Input: part model. Units: mm. Frame: model coordinates. Coordinates: 2 decimals unless noted, no trailing zeros. Write each loop counter-clockwise with the first axis right and the second up, starting at its lowest first coordinate (ties: lowest second). Pieces come first, ordered by that corner, then holes. Notation, with made-up numbers: M 80.25,-32 L 99.25,-32 A21 cw 99.25,-24 Z; hole C -5.75,-21 d3. An arc over 180 degrees is marked long. Answer as a JSON object with one key per item and string values. Group by question number.
from build123d import *

# Parameters (mm, degrees)
BOSS_EXTRUDE1_DEPTH = 5
SKETCH4_W           = 27
SKETCH4_H           = 24
SKETCH4_W_2         = 24
CUT_EXTRUDE1_DEPTH  = 6
SKETCH5_R           = 3
CUT_EXTRUDE2_DEPTH  = 44
SKETCH6_R           = 3
CUT_EXTRUDE3_DEPTH  = 70
SKETCH7_R           = 3
CUT_EXTRUDE4_DEPTH  = 95


with BuildPart() as part:
    # Sketch1 → Boss-Extrude1 (new body)
    with BuildSketch(Plane(origin=(0, 0, 0), x_dir=(1, 0, 0), z_dir=(0, 1, 0))):
        with BuildLine():
            Line((0, 0), (0, 160))
            ThreePointArc((0, 160), (80, 209.178296965), (160, 160))
            Line((160, 160), (160, 0))
            ThreePointArc((160, 0), (80, -49.178296965), (0, 0))
        make_face()
    extrude(amount=BOSS_EXTRUDE1_DEPTH)

    # Sketch4 → Cut-Extrude1 (cut)
    with BuildSketch(Plane(origin=(0, 5, 0), x_dir=(1, 0, 0), z_dir=(0, 1, 0))):
        with BuildLine():
            Line((21.873652217, 157.907743676), (47, 157.907743676))
            Line((47, 157.907743676), (47, 180.865592736))
            ThreePointArc((47, 180.865592736), (33.013102641, 170.944870409), (21.873652217, 157.907743676))
        make_face()
        with BuildLine():
            Line((53, 157.907743676), (77, 157.907743676))
            Line((77, 157.907743676), (77, 189.11366611))
            ThreePointArc((77, 189.11366611), (64.76062681, 187.490880041), (53, 183.732775763))
            Line((53, 183.732775763), (53, 157.907743676))
        make_face()
        with BuildLine():
            Line((83, 157.907743676), (107, 157.907743676))
            Line((107, 157.907743676), (107, 183.732775763))
            ThreePointArc((107, 183.732775763), (95.23937319, 187.490880041), (83, 189.11366611))
            Line((83, 189.11366611), (83, 157.907743676))
        make_face()
        with BuildLine():
            Line((113, 157.907743676), (138.126347783, 157.907743676))
            ThreePointArc((138.126347783, 157.907743676), (126.986897359, 170.944870409), (113, 180.865592736))
            Line((113, 180.865592736), (113, 157.907743676))
        make_face()
        with Locations((126.5, 139.907743676)):
            Rectangle(SKETCH4_W, SKETCH4_H)
        with Locations((95, 139.907743676)):
            Rectangle(SKETCH4_W_2, SKETCH4_H)
        with Locations((65, 139.907743676)):
            Rectangle(SKETCH4_W_2, SKETCH4_H)
        with Locations((33.5, 139.907743676)):
            Rectangle(SKETCH4_W, SKETCH4_H)
        with Locations((33.5, 109.907743676)):
            Rectangle(SKETCH4_W, SKETCH4_H)
        with Locations((65, 109.907743676)):
            Rectangle(SKETCH4_W_2, SKETCH4_H)
        with Locations((95, 109.907743676)):
            Rectangle(SKETCH4_W_2, SKETCH4_H)
        with Locations((126.5, 109.907743676)):
            Rectangle(SKETCH4_W, SKETCH4_H)
        with Locations((126.5, 79.907743676)):
            Rectangle(SKETCH4_W, SKETCH4_H)
        with Locations((95, 79.907743676)):
            Rectangle(SKETCH4_W_2, SKETCH4_H)
        with Locations((65, 79.907743676)):
            Rectangle(SKETCH4_W_2, SKETCH4_H)
        with Locations((33.5, 79.907743676)):
            Rectangle(SKETCH4_W, SKETCH4_H)
        with Locations((33.5, 49.907743676)):
            Rectangle(SKETCH4_W, SKETCH4_H)
        with Locations((65, 49.907743676)):
            Rectangle(SKETCH4_W_2, SKETCH4_H)
        with Locations((95, 49.907743676)):
            Rectangle(SKETCH4_W_2, SKETCH4_H)
        with Locations((126.5, 49.907743676)):
            Rectangle(SKETCH4_W, SKETCH4_H)
        with Locations((126.5, 19.907743676)):
            Rectangle(SKETCH4_W, SKETCH4_H)
        with Locations((95, 19.907743676)):
            Rectangle(SKETCH4_W_2, SKETCH4_H)
        with Locations((65, 19.907743676)):
            Rectangle(SKETCH4_W_2, SKETCH4_H)
        with Locations((33.5, 19.907743676)):
            Rectangle(SKETCH4_W, SKETCH4_H)
        with BuildLine():
            Line((47, -20.865592736), (47, 1.907743676))
            Line((47, 1.907743676), (21.995929992, 1.907743676))
            ThreePointArc((21.995929992, 1.907743676), (33.09486806, -11.019460066), (47, -20.865592736))
        make_face()
        with BuildLine():
            Line((77, -29.11366611), (77, 1.907743676))
            Line((77, 1.907743676), (53, 1.907743676))
            Line((53, 1.907743676), (53, -23.732775763))
            ThreePointArc((53, -23.732775763), (64.76062681, -27.490880041), (77, -29.11366611))
        make_face()
        with BuildLine():
            Line((107, -23.732775763), (107, 1.907743676))
            Line((107, 1.907743676), (83, 1.907743676))
            Line((83, 1.907743676), (83, -29.11366611))
            ThreePointArc((83, -29.11366611), (95.23937319, -27.490880041), (107, -23.732775763))
        make_face()
        with BuildLine():
            ThreePointArc((113, -20.865592736), (126.90513194, -11.019460066), (138.004070008, 1.907743676))
            Line((138.004070008, 1.907743676), (113, 1.907743676))
            Line((113, 1.907743676), (113, -20.865592736))
        make_face()
    extrude(amount=-CUT_EXTRUDE1_DEPTH, mode=Mode.SUBTRACT)

    # Sketch5 → Cut-Extrude2 (cut)
    with BuildSketch(Plane(origin=(0, 5, 0), x_dir=(1, 0, 0), z_dir=(0, 1, 0))):
        with Locations(Location((10, 37.5, 0), (0, 0, 270))):
            Circle(SKETCH5_R)
        with Locations(Location((150, 37.5, 0), (0, 0, 270))):
            Circle(SKETCH5_R)
        with Locations(Location((150, 122.5, 0), (0, 0, 270))):
            Circle(SKETCH5_R)
        with Locations(Location((10, 122.5, 0), (0, 0, 270))):
            Circle(SKETCH5_R)
    extrude(amount=-CUT_EXTRUDE2_DEPTH, mode=Mode.SUBTRACT)

    # Sketch6 → Cut-Extrude3 (cut)
    with BuildSketch(Plane(origin=(0, 5, 0), x_dir=(1, 0, 0), z_dir=(0, 1, 0))):
        with Locations(Location((9.88568101, 144.5, 0), (0, 0, 270))):
            Circle(SKETCH6_R)
        with Locations((9.88568101, 122.5)):
            Circle(SKETCH6_R)
        with Locations(Location((10, 15.5, 0), (0, 0, 270))):
            Circle(SKETCH6_R)
        with Locations(Location((150, 144.5, 0), (0, 0, 270))):
            Circle(SKETCH6_R)
        with Locations(Location((150, 15.5, 0), (0, 0, 270))):
            Circle(SKETCH6_R)
    extrude(amount=-CUT_EXTRUDE3_DEPTH, mode=Mode.SUBTRACT)

    # Sketch7 → Cut-Extrude4 (cut)
    with BuildSketch(Plane(origin=(0, 5, 0), x_dir=(1, 0, 0), z_dir=(0, 1, 0))):
        with Locations(Location((10, 166, 0), (0, 0, 270))):
            Circle(SKETCH7_R)
        with Locations(Location((150, 166, 0), (0, 0, 270))):
            Circle(SKETCH7_R)
        with Locations(Location((150, -6, 0), (0, 0, 270))):
            Circle(SKETCH7_R)
        with Locations(Location((10, -6, 0), (0, 0, 270))):
            Circle(SKETCH7_R)
    extrude(amount=-CUT_EXTRUDE4_DEPTH, mode=Mode.SUBTRACT)


solid = part.part
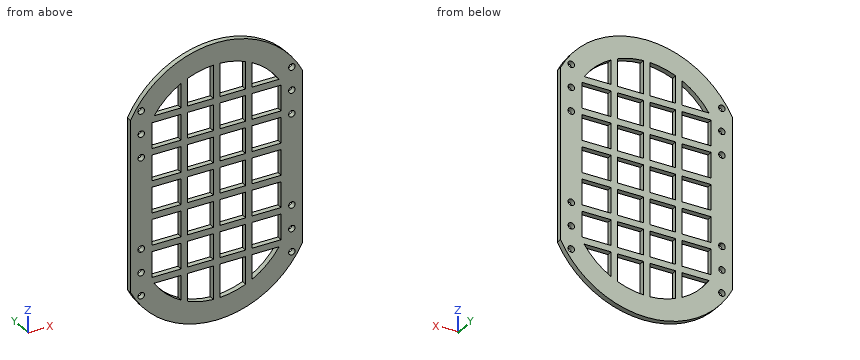
Q1. Pin query (flat end, axial travel): pin 1 Ø1.5 at (x, y) = (29, 2.5) entering from -Z; pin 2 Ø1.5 at (x, y) = (33.5, 3) entering from +Z; pin 3 Ø2.5 at (x, y) = (71, 2) entering from +Z. Return the tip coordinate at first contact, or that it passes through.
Q2. Section B-B, the plane z = -15.5. Return the cut outline in (x, y), and give its area (3 significant figures).
Q3. Section D-D, the plane x = 150. Return the cut outline in (y, z).
Q4. Line query: line 1 (X direction, y = 3.4, z = -37.5); line 2 (X direction, y = 2.45, z = -83); line 3 (X direction, y = 3, z = -1). Output: solid intervals per line, ascending. Write a range as from..to.
Q5. Section C-C, the plane x = 72. State how many separate pieces and enclosed holes the cut face has, and give its area (3 significant figures).
Q6. Section A-A, the plane z = -72.5. Return the cut outline in (x, y).
Filled in:
{
 "1": {"pin 1": "z = -193.77", "pin 2": "z = 36.63", "pin 3": "z = 48.84"},
 "2": {"outline": "M 0,0 L 7,0 L 7,5 L 0,5 Z; M 13,0 L 20,0 L 20,5 L 13,5 Z; M 47,0 L 53,0 L 53,5 L 47,5 Z; M 77,0 L 83,0 L 83,5 L 77,5 Z; M 107,0 L 113,0 L 113,5 L 107,5 Z; M 140,0 L 147,0 L 147,5 L 140,5 Z; M 153,0 L 160,0 L 160,5 L 153,5 Z", "area": "230 mm^2"},
 "3": {"outline": "M 0,-175.54 L 5,-175.54 L 5,-169 L 0,-169 Z; M 0,-163 L 5,-163 L 5,-147.5 L 0,-147.5 Z; M 0,-141.5 L 5,-141.5 L 5,-125.5 L 0,-125.5 Z; M 0,-119.5 L 5,-119.5 L 5,-40.5 L 0,-40.5 Z; M 0,-34.5 L 5,-34.5 L 5,-18.5 L 0,-18.5 Z; M 0,-12.5 L 5,-12.5 L 5,3 L 0,3 Z; M 0,9 L 5,9 L 5,15.54 L 0,15.54 Z"},
 "4": {"line 1": "0..7, 13..147, 153..160", "line 2": "0..20, 47..53, 77..83, 107..113, 140..160", "line 3": "0..22.61, 47..53, 77..83, 107..113, 137.39..160"},
 "5": {"separate pieces": "8", "enclosed holes": "0", "area": "381 mm^2"},
 "6": {"outline": "M 0,0 L 20,0 L 20,5 L 0,5 Z; M 47,0 L 53,0 L 53,5 L 47,5 Z; M 77,0 L 83,0 L 83,5 L 77,5 Z; M 107,0 L 113,0 L 113,5 L 107,5 Z; M 140,0 L 160,0 L 160,5 L 140,5 Z"}
}
